Autodesk Inventor part; units mm, degrees
ref_plane "YZ Plane" through (0, 0, 0) normal (1, 0, 0) x (0, 1, 0)
ref_plane "XZ Plane" through (0, 0, 0) normal (0, 1, 0) x (-1, 0, 0)
ref_plane "XY Plane" through (0, 0, 0) normal (0, 0, 1) x (1, 0, 0)
sketch "Sketch1" plane through (0, 0, 0) normal (1, 0, 0) x (0, 1, 0)
  line L0 (0, 0) -> (20.32, 0)
  line L1 (20.32, 0) -> (20.32, 20.32)
  line L2 (20.32, 20.32) -> (0, 20.32)
  line L3 (0, 20.32) -> (0, 0)
  dimension "d0" = 20.32
  dimension "d1" = 20.32
extrude "Extrusion1" add sketch "Sketch1" along normal blind 7.62
sketch "Sketch2" plane through (7.62, 0, 0) normal (1, 0, 0) x (0, 0, -1)
  circle A0 centre (-10.16, 10.16) radius 9.525
  point P0 (0, 0)
  dimension "d4" = 19.05
extrude "Extrusion2" add sketch "Sketch2" along normal blind 12.7
fillet "Fillet1" radius 5.588 4 edges at (3.81, 20.32, 0) (3.81, 0, 0) (3.81, 0, 20.32) (3.81, 20.32, 20.32)
sketch "Sketch3" plane through (20.32, 10.16, 10.16) normal (1, 0, 0) x (0, 0, -1)
  circle A0 centre (0, 0) radius 9.525
  circle A1 centre (0, 0) radius 9.125
  point P0 (10.16, -10.16)
  dimension "d8" = 18.25
extrude "Extrusion3" cut sketch "Sketch3" against normal blind 2.72
sketch "Sketch4" plane through (20.32, 10.16, 10.16) normal (1, 0, 0) x (0, 0, -1)
  circle A0 centre (0, 0) radius 9.525
  point P0 (10.16, -10.16)
extrude "Extrusion4" add sketch "Sketch4" against normal blind 1.5
sketch "Sketch5" plane through (0, 0, 0) normal (-1, 0, 0) x (0, 0, 1)
  circle A0 centre (10.16, 10.16) radius 9.125
  circle A1 centre (10.16, 10.16) radius 4
  point P0 (0, 0)
  dimension "d13" = 8
extrude "Extrusion5" cut sketch "Sketch5" against normal blind 25 contours A1
sketch "Sketch6" plane through (0, 0, 0) normal (-1, 0, 0) x (0, 0, 1)
  circle A0 centre (10.16, 10.16) radius 4
  circle A1 centre (10.16, 10.16) radius 4
  circle A2 centre (10.16, 10.16) radius 5
  point P0 (0, 0)
  dimension "d16" = 10
extrude "Extrusion6" add sketch "Sketch6" along normal blind 5
fillet "Fillet2" radius 2 1 edges at (0, 10.16, 5.16)
properties part number "_3DPrint"
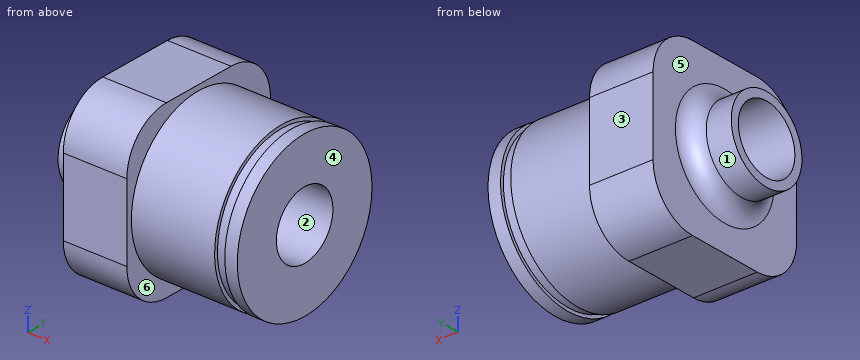
The model under review builds one solid part; all positions refer to its coordinate system, in mm. Face numbers are marked on the shaded views. A direction names the side the tool comes from. Round coordinates to 2 decimals unless told otherwise and drop trailing zeros. Write each loop counter-clockwise with the first axis right and the second up, starting at its lowest first coordinate (ties: lowest second). Pieces come first, ordered by that corner, then holes. Notation, with made-up numbers: (60, -18.5) -> (67, -18.5) arc R19 cw to (67, 17.5) -> close; hole circle Ø10 at (-33.5, -6). An arc over 180 degrees is marked (long way). Answer as a JSON object with one key per item and string values.
1. The part is to be moulded in two halves that separate along Z. For the marked faces 1, 2 and 3, say which applies: pulls with the +Z half, pulls with the -Z half, needs draft (parallel to the pull), parting line crosses it, or undercut.
Results found:
{"face 1": "parting line crosses it", "face 2": "undercut", "face 3": "needs draft"}
2. We need section A-A on x = 1.5. State the section outline as (y, z) points.
Results found:
{"outline": "(0, 5.59) arc R5.59 ccw to (5.59, 0) -> (14.73, 0) arc R5.59 ccw to (20.32, 5.59) -> (20.32, 14.73) arc R5.59 ccw to (14.73, 20.32) -> (5.59, 20.32) arc R5.59 ccw to (0, 14.73) -> close; hole circle Ø8 at (10.16, 10.16)"}
3. To check wall thickness, follow line 1 along X through (y, z) = (15.5, 2.5); line 2 along Y through (x, z) = (14.5, 10.16) (3 decimals); line 3 along Y through (x, z) = (5, 10.16). State the ranges of each line that lie inside material, in increasing order.
Results found:
{"line 1": "x = 0 to 17.6, 18.82 to 20.32", "line 2": "y = 0.635 to 6.16, 14.16 to 19.685", "line 3": "y = 0 to 6.16, 14.16 to 20.32"}
4. Clearance check with flat-ended pins moving along their axes: pin 1 (6 mm diameter, centred on x = 16, z = 2.5, fed in from -Y); pin 2 (7 mm diameter, centred on y = 10.16, z = 10.16, fed in from +X); pin 3 (3 mm diameter, centred on x = 11.5, z = 9.5, fed in from +Y) (3 decimals); pin 4 (4 mm diameter, centred on x = 1, z = 2.5, fed in from +Y). State where each tip first meets the part, or that it passes through.
Results found:
{"pin 1": "stops at y = 1.85", "pin 2": "passes through", "pin 3": "stops at y = 19.685", "pin 4": "stops at y = 20.21"}
5. We need section D-D on y = 2.25. State the section outline as (x, z) points, and give its area (3 significant figures).
Results found:
{"outline": "(0, 1.11) -> (7.62, 1.11) -> (7.62, 4.85) -> (17.6, 4.85) -> (17.6, 5.61) -> (18.82, 5.61) -> (18.82, 4.85) -> (20.32, 4.85) -> (20.32, 15.47) -> (18.82, 15.47) -> (18.82, 14.71) -> (17.6, 14.71) -> (17.6, 15.47) -> (7.62, 15.47) -> (7.62, 19.21) -> (0, 19.21) -> close", "area": "271 mm^2"}
6. Machinability: for the marked faces 4, 5 and 6, which of the approach directions +Z, -Z, +X, -X, +Y, -Y give a long, thin tool a straight path to every point of the face, cutting with its end or side? Answer none if there is none.
Results found:
{"face 4": "+Z, -Z, +X, +Y, -Y", "face 5": "-X", "face 6": "+X"}
7. We need section B-B on y = 10.16. State the section outline as (x, z) points (3 decimals), and give its area (3 significant figures).
Results found:
{"outline": "(-5, 5.16) -> (-2, 5.16) arc R2 cw to (0, 3.16) -> (0, 0) -> (7.62, 0) -> (7.62, 0.635) -> (17.6, 0.635) -> (17.6, 1.035) -> (18.82, 1.035) -> (18.82, 0.635) -> (20.32, 0.635) -> (20.32, 6.16) -> (-5, 6.16) -> close; (-5, 14.16) -> (20.32, 14.16) -> (20.32, 19.685) -> (18.82, 19.685) -> (18.82, 19.285) -> (17.6, 19.285) -> (17.6, 19.685) -> (7.62, 19.685) -> (7.62, 20.32) -> (0, 20.32) -> (0, 17.16) arc R2 cw to (-2, 15.16) -> (-5, 15.16) -> close", "area": "245 mm^2"}
